The listing builds one solid part. Answer for the finished solid, in the listing's coordinates (mm). Face numbers are marked on the shaded views. A direction names the side the tool comes from. Give positions to 0.01 mm unless a question says otherwise; leave off trailing zeros. Loops run counter-clockwise (first coordinate to the right, second up) from the corner with the lowest first, then second, coordinate; pieces in that order, holes last. Notation, with made-up numbers: (81.5, 35) - (123.5, 35) arc R5 ccw to (123.5, 39) - close; hole circle Ø5 at (-35.75, 78.5). An arc over 180 degrees is marked (long way). Answer as CSV lines item,"result". Start each with the question number.
1) A cutting plane is placed at A-A (z = 6). Give the number of separate pieces and of enclosed holes in the cut face, and give its area (3 significant figures).
2) Find the intervals of material crossed by line 1 along Z through (x, y) = (0, 6.25); line 2 along Y through (x, z) = (1.5, 0); line 3 along Y through (x, z) = (-35, -13), in increasing order.
3) A cutting plane is placed at B-B (y = 21.5). Determine the outline of the cut face in (x, z), and give its area (3 significant figures).
4) Flat-ended cylindrical pins translate along their axes: pin 1 (10 mm diameter, centred on y = 28, z = 10.5, fed in from -X); pin 2 (4 mm diameter, centred on x = 10.5, z = 2.5, fed in from +Y); pin 3 (4 mm diameter, centred on x = -11.5, z = -4.5, fed in from +Y). Find the tip coordinate at first contact, or state that the pin passes through.
5) For the marked faces 1 and 2, determine the directions among +Z, -Z, +X, -X, +Y, -Y from which every point of the face is accessible in a straight line to the end or side of a thin tool.
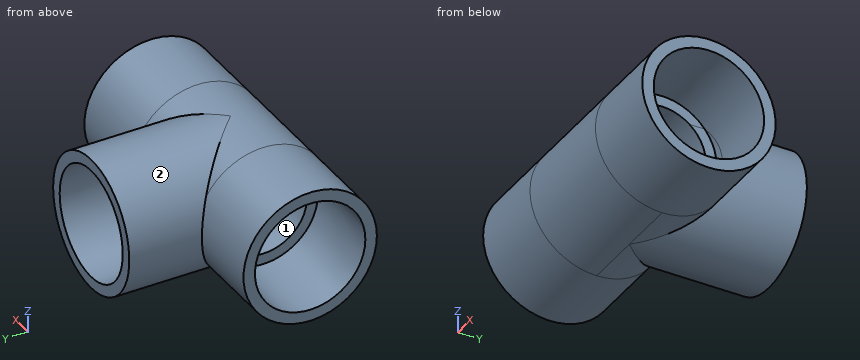
```python
from build123d import *

# Parameters (mm, degrees)
SKETCH4_R           = 20.3327
BOSS_EXTRUDE1_DEPTH = 34.9504
SKETCH5_R           = 20.3327
BOSS_EXTRUDE2_DEPTH = 17.4752


with BuildPart() as part:
    # Sketch1 → Revolve1 (revolve)
    with BuildSketch(Plane.XY):
        Polygon((-42.4942, -20.3327), (-17.4752, -20.3327), (-17.4752, -16.637), (-42.4942, -16.8275), align=None)
        Polygon((42.4942, -16.8275), (17.4752, -16.637), (17.4752, -20.3327), (42.4942, -20.3327), align=None)
    revolve(axis=Axis((-42.4942, 0, 0), (1, 0, 0)))



with BuildPart() as body_2:
    # Sketch2 → Revolve2 (revolve)
    with BuildSketch(Plane.XY):
        Polygon((16.8275, 42.4942), (16.637, 17.4752), (20.3327, 17.4752), (20.3327, 42.4942), align=None)
    revolve(axis=Axis((0, 0, 0), (0, 1, 0)))


with BuildPart() as part_1:
    add(part.part)

    add(body_2.part)  # Boss-Extrude1 merges body 2
    # Sketch4 → Boss-Extrude1 (add)
    with BuildSketch(Plane(origin=(-17.4752, 0, 0), x_dir=(0, 0, -1), z_dir=(1, 0, 0))):
        Circle(SKETCH4_R)
    extrude(amount=BOSS_EXTRUDE1_DEPTH)

    # Sketch5 → Boss-Extrude2 (add)
    with BuildSketch(Plane.XZ.offset(-17.4752)):
        Circle(SKETCH5_R)
    extrude(amount=BOSS_EXTRUDE2_DEPTH)

    # Sketch6 → Cut-Revolve1 (revolve, cut)
    with BuildSketch(Plane.XY):
        Polygon((-42.4942, -16.8275), (-17.4752, -16.637), (-17.4752, -13.3223), (17.4752, -13.3223), (17.4752, -16.637), (42.4942, -16.8275), (42.4942, 0), (-42.4942, 0), align=None)
    revolve(axis=Axis((42.4942, 0, 0), (-1, 0, 0)), mode=Mode.SUBTRACT)

    # Sketch7 → Cut-Revolve2 (revolve, cut)
    with BuildSketch(Plane.XY):
        Polygon((16.8275, 42.4942), (16.637, 17.4752), (13.3223, 17.4752), (13.3223, 0), (0, 0), (0, 42.4942), align=None)
    revolve(axis=Axis((0, 0, 0), (0, 1, 0)), mode=Mode.SUBTRACT)


solid = part_1.part
```
Ans:
1,separate pieces,"3"
1,enclosed holes,"0"
1,area,"890 mm2"
2,line 1,"-20.33 to -13.32, 13.32 to 20.33"
2,line 2,"-20.33 to -13.32"
2,line 3,"-15.63 to -10.59, 10.59 to 15.63"
3,outline,"circle Ø40.67 at (0, 0); hole circle Ø33.34 at (0, 0)"
3,area,"426 mm2"
4,pin 1,"x = -19.57"
4,pin 2,"y = -12.54"
4,pin 3,"y = 17.48"
5,face 1,"+X, -X"
5,face 2,"+Y"
